The listing builds one solid part. Answer for the finished solid, in the listing's coordinates (mm). Face numbers are marked on the shaded views. A direction names the side the tool comes from. Coordinates: 2 decimals unless noted, no trailing zeros. Order: outer loops, then holes, each group sorted by start corner. A loop starts at its lowest first (then second) coordinate and runs counter-clockwise, first axis right, second up. Notation, with made-up numbers: (16, 55) -> (68, 55) arc R38 cw to (68, 94) -> close; hole circle Ø3 at (-15.5, -19). An arc over 180 degrees is marked (long way). Return JSON: item names as keys, results as strings.
Autodesk Inventor part; units mm, degrees
ref_plane "YZ Plane" through (0, 0, 0) normal (1, 0, 0) x (0, 1, 0)
ref_plane "XZ Plane" through (0, 0, 0) normal (0, 1, 0) x (-1, 0, 0)
ref_plane "XY Plane" through (0, 0, 0) normal (0, 0, 1) x (1, 0, 0)
sketch "Sketch1" plane through (0, 0, 0) normal (0, 0, 1) x (1, 0, 0)
  circle A0 centre (0, 0) radius 4.6
  dimension "d0" = 9.2
extrude "Extrusion1" add sketch "Sketch1" along normal blind 4.6
sketch "Sketch2" plane through (0, 0, 0) normal (0, 0, -1) x (-1, 0, 0)
  circle A0 centre (0, 0) radius 2.6
  dimension "d3" = 5.2
extrude "Extrusion2" cut sketch "Sketch2" against normal blind 2.6
sketch "Sketch4" plane through (0, 0, 4.6) normal (0, 0, 1) x (1, 0, 0)
  line L0 (0.8, 6.5) -> (-0.8, 6.5)
  line L1 (-0.8, 6.5) -> (-0.8, -6.5)
  line L2 (-0.8, -6.5) -> (0.8, -6.5)
  line L3 (0.8, -6.5) -> (0.8, 6.5)
  line L4 (0.8, 6.5) -> (-0.8, -6.5) construction
  line L5 (-0.8, 6.5) -> (0.8, -6.5) construction
  circle A0 centre (0, 0) radius 4.6
  circle A1 centre (0, 0) radius 4.6
  point P0 (0.8, 4.5299)
  point P1 (-0.8, 4.5299)
  point P2 (-0.8, -4.5299)
  point P3 (0.8, -4.5299)
  dimension "d14" = 1.6
  dimension "d15" = 13
extrude "Extrusion4" add sketch "Sketch4" along normal blind 1 contours L3 A0 L1
properties part number "RamaKola"
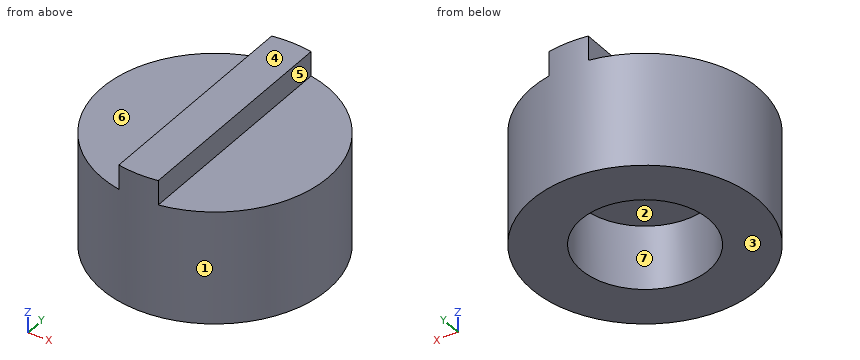
Item 1: Which of the six approach directions +Z, -Z, +X, -X, +Y, -Y give full straight-line access (tool end or side, diameter ignored) to the marked faces 4, 5, 6 and 7?
Answer list:
{"face 4": "+Z, +X, -X, +Y, -Y", "face 5": "+Z, +X, +Y, -Y", "face 6": "+Z, -X, +Y, -Y", "face 7": "-Z"}
Item 2: Determine the mould class of the marked faces 1, 2 and 3 for opening direction Y: pulls with the +Y half, pulls with the -Y half, needs draft (parallel to the pull), parting line crosses it, or undercut.
Answer list:
{"face 1": "parting line crosses it", "face 2": "undercut", "face 3": "needs draft"}
Item 3: Flat-ended cylindrical pins translate along their axes: pin 1 (4 mm diameter, centred on x = 0, y = 0.5, fed in from -Z); pin 2 (1.1 mm diameter, centred on x = -2.5, y = -2, fed in from +Z); pin 3 (0.5 mm diameter, centred on y = -1, z = 5.5, fed in from -X). Find the tip coordinate at first contact, or state that the pin passes through.
Answer list:
{"pin 1": "z = 2.6", "pin 2": "z = 4.6", "pin 3": "x = -0.8"}
Item 4: The part is cut by section D-D on z = 3.25. Determine the outline of the cut face in (x, y), plus the area to 3 significant figures.
Answer list:
{"outline": "circle Ø9.2 at (0, 0)", "area": "66.5 mm2"}
Item 5: Find the intervals of material crossed by probe 1 along Y at (x, z) = (0, 1.2); probe 2 along Z at (x, y) = (-2.75, -2); probe 3 along Z at (x, y) = (2, 0.5), in increasing order.
Answer list:
{"probe 1": "-4.6 to -2.6, 2.6 to 4.6", "probe 2": "0 to 4.6", "probe 3": "2.6 to 4.6"}
Item 6: The part is cut by section B-B on z = 2.2. Determine the outline of the cut face in (x, y), plus the area to 3 significant figures.
Answer list:
{"outline": "circle Ø9.2 at (0, 0); hole circle Ø5.2 at (0, 0)", "area": "45.2 mm2"}
Item 7: The part is cut by section A-A on y = 0. Determine the outline of the cut face in (x, z).
Answer list:
{"outline": "(-4.6, 0) -> (-2.6, 0) -> (-2.6, 2.6) -> (2.6, 2.6) -> (2.6, 0) -> (4.6, 0) -> (4.6, 4.6) -> (0.8, 4.6) -> (0.8, 5.6) -> (-0.8, 5.6) -> (-0.8, 4.6) -> (-4.6, 4.6) -> close"}
Item 8: The part is cut by section C-C on x = 0. Determine the outline of the cut face in (y, z), plus the area to 3 significant figures.
Answer list:
{"outline": "(-4.6, 0) -> (-2.6, 0) -> (-2.6, 2.6) -> (2.6, 2.6) -> (2.6, 0) -> (4.6, 0) -> (4.6, 5.6) -> (-4.6, 5.6) -> close", "area": "38.0 mm2"}
